Geometry: see drawing. Coordinates: mm, zero at the bounding-box minimum. Round coordinates to 2 decimals unless told otherwise and drop trailing zeros. Loops run counter-clockwise (first coordinate to the right, second up) from the corner with the lowest first, then second, coordinate; pieces in that order, holes last. Notation, with made-up numbers: (10.5, -12.75) - (55.5, -12.75) arc R35 cw to (55.5, 26.25) - close; hole circle Ø10 at (62.25, 1). An arc over 180 degrees is marked (long way). Write item = value, one per line. Start each with the question number.
Item 1: Line query: line 1 (X direction, y = 139, z = 2.5); line 2 (Y direction, x = 13.5, z = 1.15); line 3 (Y direction, x = 13.75, z = 1.05). Output: solid intervals per line, ascending. Write a range as from..to.
Item 2: Section B-B (y = 109.5). Return loops of the section in (x, z) (1 decimal), plus the area to 3 significant figures.
Item 3: First-contact query: pin 1 (1 mm diameter, centred on y = 33, z = 2, fed in from +X). Flat tip, straight axial feed; report the tip coordinate or a pass-through.
Item 4: Section A-A (z = 2.35). Return loops of the section in (x, y), plus the area to 3 significant figures.
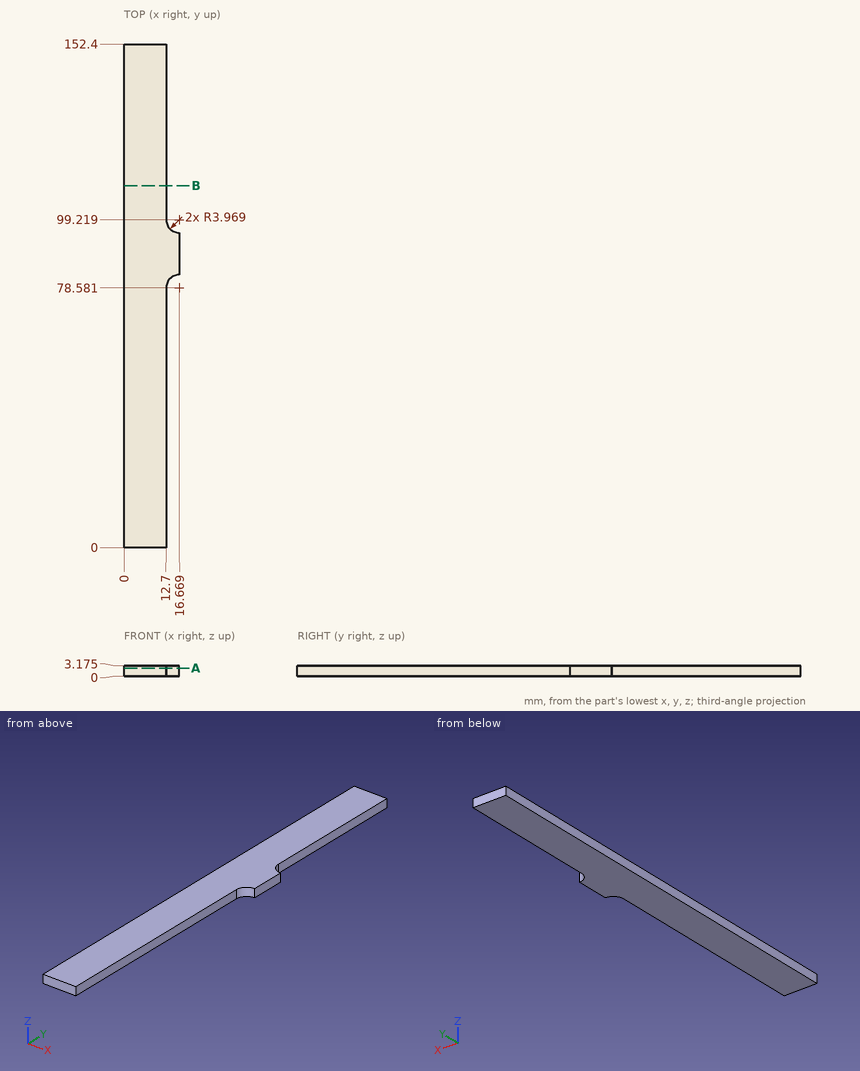
Taken from the geometry:
q1.line_1 = 0..12.7
q1.line_2 = 80.97..96.83
q1.line_3 = 81.27..96.53
q2.outline = (0, 0) - (12.7, 0) - (12.7, 3.2) - (0, 3.2) - close
q2.area = 40.3 mm^2
q3.pin_1 = 12.7
q4.outline = (0, 0) - (12.7, 0) - (12.7, 78.58) arc R3.97 cw to (16.67, 82.55) - (16.67, 95.25) arc R3.97 cw to (12.7, 99.22) - (12.7, 152.4) - (0, 152.4) - close
q4.area = 1,990 mm^2
